Input: part model. Units: mm. Frame: model coordinates. Face numbers are marked on the shaded views. A direction names the side the tool comes from. Round coordinates to 2 decimals unless told otherwise and drop trailing zeros. Loops run counter-clockwise (first coordinate to the right, second up) from the corner with the lowest first, then second, coordinate; pieces in that order, holes last. Notation, with made-up numbers: (16.25, 37) -> (66.25, 37) arc R26 cw to (66.25, 76) -> close; hole circle Ø5 at (-6, -4). An arc over 180 degrees is marked (long way). Answer as a JSON object with one key per item and string values.
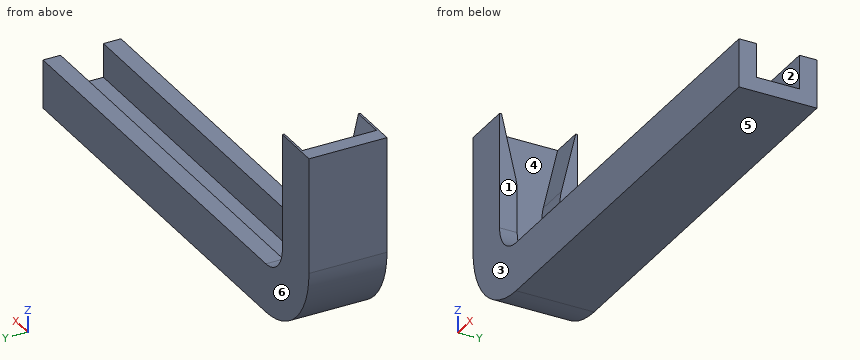
```python
from build123d import *

# Parameters (mm, degrees)
SKETCH1_W           = 50
SKETCH1_H           = 8
BOSS_EXTRUDE1_DEPTH = 20
SKETCH2_W           = 48.4
SKETCH2_H           = 4.4
CUT_EXTRUDE1_DEPTH  = 18.5
SKETCH3_W           = 45
SKETCH3_H           = 15
CUT_EXTRUDE2_DEPTH  = 18
FILLET1_R           = 6.6
FILLET2_R           = 8.1
FILLET3_R           = 3.1
CHAMFER1_SIZE       = 1.6
CHAMFER1_SIZE2      = 6.930361399
FILLET4_R           = 5


with BuildPart() as part:
    # Sketch1 → Boss-Extrude1 (new body)
    with BuildSketch(Plane.XY):
        with Locations((25, 4)):
            Rectangle(SKETCH1_W, SKETCH1_H)
    extrude(amount=BOSS_EXTRUDE1_DEPTH)

    # Sketch2 → Cut-Extrude1 (cut)
    with BuildSketch(Plane.XY.offset(20)):
        with Locations((25.8, 4.003663633)):
            Rectangle(SKETCH2_W, SKETCH2_H)
    extrude(amount=-CUT_EXTRUDE1_DEPTH, mode=Mode.SUBTRACT)

    # Sketch3 → Cut-Extrude2 (cut)
    with BuildSketch(Plane(origin=(0, 0, 0), x_dir=(-1, 0, 0), z_dir=(0, -1, 0))):
        with Locations((-27.5, -12.5)):
            Rectangle(SKETCH3_W, SKETCH3_H)
    extrude(amount=-CUT_EXTRUDE2_DEPTH, mode=Mode.SUBTRACT)

    # Fillet1
    fillet1_edges = [part.edges().sort_by_distance(p)[0] for p in [
        (1.6, 4.003663633, 1.5),
    ]]
    fillet(fillet1_edges, radius=FILLET1_R)

    # Fillet2
    fillet2_edges = [part.edges().sort_by_distance(p)[0] for p in [
        (0, 4, 0),
    ]]
    fillet(fillet2_edges, radius=FILLET2_R)

    # Fillet3
    fillet3_edges = [part.edges().sort_by_distance(p)[0] for p in [
        (5, 7.101831816, 5),
        (5, 0.901831816, 5),
    ]]
    fillet(fillet3_edges, radius=FILLET3_R)

    # Chamfer1
    chamfer1_edges = [part.edges().sort_by_distance(p)[0] for p in [
        (3.3, 1.803663633, 20),
        (3.3, 6.203663633, 20),
    ]]
    chamfer1_side = [part.faces().sort_by_distance(p)[0] for p in [
        (2.5, 7.905660189, 20),
    ]]
    chamfer(chamfer1_edges, length=CHAMFER1_SIZE, length2=CHAMFER1_SIZE2, reference=chamfer1_side[0])

    # Fillet4
    fillet4_edges = [part.edges().sort_by_distance(p)[0] for p in [
        (3.3, 1.803663633, 13.069638601),
        (3.3, 6.203663633, 13.069638601),
    ]]
    fillet(fillet4_edges, radius=FILLET4_R)


solid = part.part
```
1) Ray query, probe 1 along Y at (x, z) = (3.5, 9.5); probe 2 along Z at (x, y) = (42, 4.5); probe 3 along Z at (x, y) = (26.5, 0.5). Return the intervals inside material, ascending.
Output:
{"probe 1": "y = 0 to 1.8, 6.2 to 8", "probe 2": "z = 0 to 1.5", "probe 3": "z = 0 to 5"}
2) Section B-B, the plane y = 4. Output: boundary loops of the cut face in (x, z), plus the area to 3 significant figures.
Output:
{"outline": "(0, 8.1) arc R8.1 ccw to (8.1, 0) -> (50, 0) -> (50, 1.5) -> (8.2, 1.5) arc R6.6 cw to (1.6, 8.1) -> (1.6, 20) -> (0, 20) -> close", "area": "99.9 mm^2"}
3) Contact query for flat-ended pins moving along their axis: P1, Ø1.4, axis at x = 33, y = 1, coming from the +Z side; P2, Ø2, axis at y = 7, z = 13.5, coming from the +X side; P3, Ø10, axis at x = 20.5, z = 4.5, coming from the -Y side. Output: stop coordinate, or through.
Output:
{"P1": "stops at z = 5", "P2": "stops at x = 5", "P3": "stops at y = 0"}
4) Draft query along Y for the marked faces 4, 5 and 6. Return one class per face: +Y half, -Y half, draft (parallel to the pull), parting line (faces both ways), or undercut.
Output:
{"face 4": "undercut", "face 5": "draft", "face 6": "+Y half"}
5) Section A-A, the plane z = 11. Output: boundary loops of the cut face in (x, y).
Output:
{"outline": "(0, 0) -> (5, 0) -> (5, 1.8) -> (1.6, 1.8) -> (1.6, 6.2) -> (5, 6.2) -> (5, 8) -> (0, 8) -> close"}
6) Reachability of the marked faces 1, 2 and 3 from +Z, -Z, +X, -X, +Y, -Y: full face, straight path, thin tool, end or side. Return the list, or none.
Output:
{"face 1": "+Z, +X, +Y, -Y", "face 2": "+Z, +X", "face 3": "+Z, -Z, +X, -X, -Y"}
